Here's how the part is built. I have some questions about the finished solid (model axes, mm). Face numbers are marked on the shaded views. Round coordinates to 2 decimals unless told otherwise and drop trailing zeros. Order: outer loops, then holes, each group sorted by start corner. A loop starts at its lowest first (then second) coordinate and runs counter-clockwise, first axis right, second up. Notation, with made-up numbers: (71, -13) - (106, -13) arc R22 ccw to (106, 4) - close; hole circle Ø3 at (57, -26.75). An arc over 180 degrees is marked (long way). Answer as a JSON object with one key per item and string values.
```python
from build123d import *

# Parameters (mm, degrees)
F0_R     = 47
F1_DEPTH = 18
F2_R     = 39
F3_DEPTH = 50
F4_R     = 2.5
F5_DEPTH = 22
F6_R     = 36.831923
F7_DEPTH = 2.54


with BuildPart() as f1:
    # F0 (on Top) → F1 (new body)
    with BuildSketch(Plane.XY):
        Circle(F0_R)
    extrude(amount=F1_DEPTH)

    # F2 (on face) → F3 (join)
    with BuildSketch(Plane(origin=(0, 0, 0), x_dir=(1, 0, 0), z_dir=(0, 0, -1))):
        Circle(F2_R)
    extrude(amount=F3_DEPTH)

    # F4 (on face) → F5 (join)
    with BuildSketch(Plane(origin=(0, 0, -50), x_dir=(1, 0, 0), z_dir=(0, 0, -1))):
        with Locations((-27, 0)):
            Circle(F4_R)
        with Locations((26.999997, 0)):
            Circle(F4_R)
    extrude(amount=F5_DEPTH)

    # F6 (on face) → F7 (cut)
    with BuildSketch(Plane.XY.offset(18)):
        with Locations((0, 3.63045)):
            Circle(F6_R)
    extrude(amount=-F7_DEPTH, mode=Mode.SUBTRACT)


solid = f1.part
```
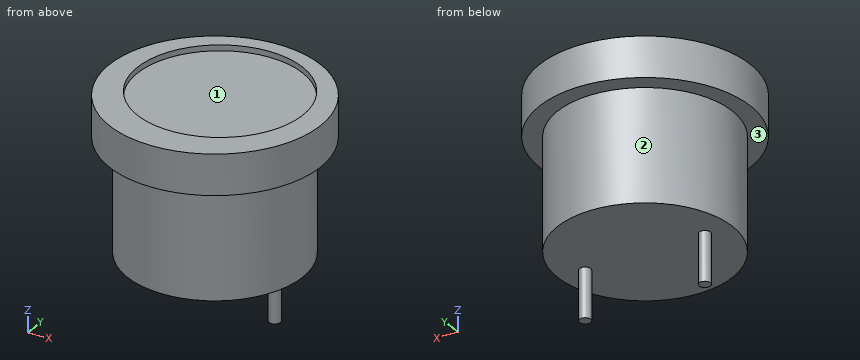
1. Imagine slicing it at C-C (z = -13). List the corners of the cut face in (x, y) for me, plus the area to 3 significant figures.
Responses:
{"outline": "circle Ø78 at (0, 0)", "area": "4,780 mm2"}
2. If I drill on L1, parallel to Y at x = 0, z = 17.4; L2, parallel to Z at x = -17, y = -12.5; L3, parallel to Z at x = 31, y = 34.5, over which ranges is the centre line in solid material (lowest first)? Write a range as [from, to].
Responses:
{"L1": "[-47, -33.2], [40.46, 47]", "L2": "[-50, 15.46]", "L3": "[0, 18]"}
3. Thinking about a two-plate mould opening in X: for the marked faces 1, 2 and 3, which applies, pulls with the +X half, pulls with the -X half, needs draft (parallel to the pull), parting line crosses it, or undercut?
Responses:
{"face 1": "undercut", "face 2": "parting line crosses it", "face 3": "needs draft"}
4. Imagine slicing it at A-A (x = 0). List the corners of the cut face in (y, z) for me.
Responses:
{"outline": "(-47, 0) - (-39, 0) - (-39, -50) - (39, -50) - (39, 0) - (47, 0) - (47, 18) - (40.46, 18) - (40.46, 15.46) - (-33.2, 15.46) - (-33.2, 18) - (-47, 18) - close"}
5. Imagine slicing it at B-B (y = 0). List the corners of the cut face in (x, z) for me.
Responses:
{"outline": "(-47, 0) - (-39, 0) - (-39, -50) - (-29.5, -50) - (-29.5, -72) - (-24.5, -72) - (-24.5, -50) - (24.5, -50) - (24.5, -72) - (29.5, -72) - (29.5, -50) - (39, -50) - (39, 0) - (47, 0) - (47, 18) - (36.65, 18) - (36.65, 15.46) - (-36.65, 15.46) - (-36.65, 18) - (-47, 18) - close"}
6. For P1, Ø12, axis at y = 21, z = -49.5, coming from the +X side; P2, Ø12, axis at x = 11.5, z = -52.5, coming from the -Y side; P3, Ø6, axis at y = -10, z = -22.5, coming from the -X side, each with a flat end and sliding along its axis, tell me the tip position at first contact or that it passes through.
Responses:
{"P1": "x = 36", "P2": "y = -38.53", "P3": "x = -38.37"}
7. Imagine slicing it at D-D (x = 22). List the corners of the cut face in (y, z) for me, plus the area to 3 significant figures.
Responses:
{"outline": "(-41.53, 0) - (-32.2, 0) - (-32.2, -50) - (32.2, -50) - (32.2, 0) - (41.53, 0) - (41.53, 18) - (33.17, 18) - (33.17, 15.46) - (-25.91, 15.46) - (-25.91, 18) - (-41.53, 18) - close", "area": "4,570 mm2"}
